Input: part model. Units: mm. Frame: model coordinates. Face numbers are marked on the shaded views. A direction names the side the tool comes from. Round coordinates to 2 decimals unless told otherwise and drop trailing zeros. Loops run counter-clockwise (first coordinate to the right, second up) from the corner with the lowest first, then second, coordinate; pieces in that order, holes last. Notation, with made-up numbers: (22.25, 78.25) -> (64.25, 78.25) arc R27 cw to (64.25, 108.25) -> close; hole circle Ø4 at (61, 38.5). An arc over 180 degrees is marked (long way). One line per question, with ' | ' between items. Start each with the question number.
Q1. Cut plane C-C on x = 1. Return loops of the section in (y, z), and give its area (4 significant figures).
Q2. Material intervals for L1, parallel to X at y = 1.15, z = 7.05; L2, parallel to Z at x = 3.5, y = 1.55; L3, parallel to X at y = 3.2, z = -4.5, sorted ascending.
Q3. Cut plane D-D on z = 2.75. Return loops of the section in (x, y).
Q4. Cut plane A-A on y = 4. Return loops of the section in (x, z).
Q5. Cut plane B-B on z = 7.05. Return loops of the section in (x, y).
Q6. Access query for the marked faces 1, 2 and 3. Directions: +Z, -Z, +X, -X, +Y, -Y. A direction counts if a zero-diameter tool reaches every point of the face in a straight line with its end or side. Return the directions, or none.
Q7. Contact query for flat-ended pins moving along their axis: P1, Ø1.5, axis at y = 2.5, z = -2.5, coming from the +X side; P2, Ø1, axis at x = 7.5, z = 8, coming from the -Y side; P3, Ø0.8, axis at y = 3.5, z = 4, coming from the +X side; P4, Ø1.2, axis at y = 3.5, z = -0.5, coming from the -X side. Output: stop coordinate, or through.
Q8. Mould query, pull axis Z, two halves, no side actions, for the marked faces 4, 5, 6 and 7. Classes: pulls with the +Z half, pulls with the -Z half, needs draft (parallel to the pull), parting line crosses it, or undercut.
from build123d import *

# Parameters (mm, degrees)
SKETCH1_W           = 24.6
SKETCH1_H           = 20.1
BOSS_EXTRUDE1_DEPTH = 1.5
SKETCH2_W           = 24.6
SKETCH2_H           = 20.1
SKETCH2_W_2         = 22.1
SKETCH2_H_2         = 17.6
BOSS_EXTRUDE2_DEPTH = 3
SKETCH4_R           = 1.6
BOSS_EXTRUDE4_DEPTH = 2
SKETCH8_W           = 3.5
SKETCH8_H           = 8.1
BOSS_EXTRUDE5_DEPTH = 2


with BuildPart() as part:
    # Sketch1 → Boss-Extrude1 (new body)
    with BuildSketch(Plane(origin=(0, 0, 0), x_dir=(1, 0, 0), z_dir=(0, 1, 0))):
        Rectangle(SKETCH1_W, SKETCH1_H)
    extrude(amount=BOSS_EXTRUDE1_DEPTH)

    # Sketch2 → Boss-Extrude2 (add)
    with BuildSketch(Plane(origin=(0, 1.5, 0), x_dir=(1, 0, 0), z_dir=(0, 1, 0))):
        Rectangle(SKETCH2_W, SKETCH2_H)
        Rectangle(SKETCH2_W_2, SKETCH2_H_2, mode=Mode.SUBTRACT)
    extrude(amount=BOSS_EXTRUDE2_DEPTH)

    # Sketch4 → Boss-Extrude4 (add)
    # profile 1 of 4: a face of its own
    with BuildSketch(Plane(origin=(0, 0, 0), x_dir=(1, 0, 0), z_dir=(0, 1, 0))):
        with BuildLine():
            Line((15.8, 10.05), (12.3, 10.05))
            Line((12.3, 10.05), (12.3, 4.05))
            Line((12.3, 4.05), (15.8, 4.05))
            ThreePointArc((15.8, 4.05), (18.8, 7.05), (15.8, 10.05))
        make_face()
        with Locations(Location((15.8, 7.05, 0), (0, 0, 270))):
            Circle(SKETCH4_R, mode=Mode.SUBTRACT)
    # profile 2 of 4: a face of its own
    with BuildSketch(Plane(origin=(0, 0, 0), x_dir=(1, 0, 0), z_dir=(0, 1, 0))):
        with BuildLine():
            Line((-15.8, 4.05), (-12.3, 4.05))
            Line((-12.3, 4.05), (-12.3, 10.05))
            Line((-12.3, 10.05), (-15.8, 10.05))
            ThreePointArc((-15.8, 10.05), (-18.8, 7.05), (-15.8, 4.05))
        make_face()
        with Locations(Location((-15.8, 7.05, 0), (0, 0, 90))):
            Circle(SKETCH4_R, mode=Mode.SUBTRACT)
    # profile 3 of 4: a face of its own
    with BuildSketch(Plane(origin=(0, 0, 0), x_dir=(1, 0, 0), z_dir=(0, 1, 0))):
        with BuildLine():
            Line((15.8, -4.05), (12.3, -4.05))
            Line((12.3, -4.05), (12.3, -10.05))
            Line((12.3, -10.05), (15.8, -10.05))
            ThreePointArc((15.8, -10.05), (18.8, -7.05), (15.8, -4.05))
        make_face()
        with Locations(Location((15.8, -7.05, 0), (0, 0, 90))):
            Circle(SKETCH4_R, mode=Mode.SUBTRACT)
    # profile 4 of 4: a face of its own
    with BuildSketch(Plane(origin=(0, 0, 0), x_dir=(1, 0, 0), z_dir=(0, 1, 0))):
        with BuildLine():
            Line((-15.8, -10.05), (-12.3, -10.05))
            Line((-12.3, -10.05), (-12.3, -4.05))
            Line((-12.3, -4.05), (-15.8, -4.05))
            ThreePointArc((-15.8, -4.05), (-18.8, -7.05), (-15.8, -10.05))
        make_face()
        with Locations(Location((-15.8, -7.05, 0), (0, 0, 270))):
            Circle(SKETCH4_R, mode=Mode.SUBTRACT)
    extrude(amount=BOSS_EXTRUDE4_DEPTH)

    # Sketch8 → Boss-Extrude5 (add, through all)
    with BuildSketch(Plane(origin=(0, 2, 0), x_dir=(1, 0, 0), z_dir=(0, 1, 0))):
        with Locations((-14.05, 0)):
            Rectangle(SKETCH8_W, SKETCH8_H)
        with Locations((14.05, 0)):
            Rectangle(SKETCH8_W, SKETCH8_H)
    extrude(amount=-BOSS_EXTRUDE5_DEPTH)


solid = part.part
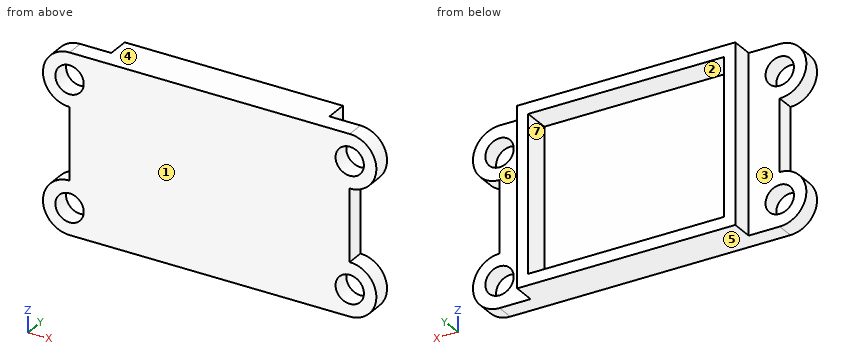
Results:
1) outline: (0, -10.05) -> (4.5, -10.05) -> (4.5, -8.8) -> (1.5, -8.8) -> (1.5, 8.8) -> (4.5, 8.8) -> (4.5, 10.05) -> (0, 10.05) -> close | area: 37.65 mm^2
2) L1: -18.8 to -17.4, -14.2 to 14.2, 17.4 to 18.8 | L2: -10.05 to -8.8, 8.8 to 10.05 | L3: -12.3 to -11.05, 11.05 to 12.3
3) outline: (-15.8, 0) -> (15.8, 0) -> (15.8, 2) -> (12.3, 2) -> (12.3, 4.5) -> (11.05, 4.5) -> (11.05, 1.5) -> (-11.05, 1.5) -> (-11.05, 4.5) -> (-12.3, 4.5) -> (-12.3, 2) -> (-15.8, 2) -> close
4) outline: (-12.3, -10.05) -> (12.3, -10.05) -> (12.3, 10.05) -> (-12.3, 10.05) -> close; hole (-11.05, -8.8) -> (11.05, -8.8) -> (11.05, 8.8) -> (-11.05, 8.8) -> close
5) outline: (-18.8, 0) -> (-17.4, 0) -> (-17.4, 2) -> (-18.8, 2) -> close; (-14.2, 0) -> (14.2, 0) -> (14.2, 2) -> (12.3, 2) -> (12.3, 4.5) -> (11.05, 4.5) -> (11.05, 1.5) -> (-11.05, 1.5) -> (-11.05, 4.5) -> (-12.3, 4.5) -> (-12.3, 2) -> (-14.2, 2) -> close; (17.4, 0) -> (18.8, 0) -> (18.8, 2) -> (17.4, 2) -> close
6) face 1: +Z, -Z, +X, -X, -Y | face 2: +Y | face 3: +Z, -Z, -X, +Y
7) P1: x = 15.8 | P2: y = 0 | P3: x = 12.3 | P4: x = -12.3
8) face 4: pulls with the +Z half | face 5: pulls with the -Z half | face 6: needs draft | face 7: undercut
